Input: part model. Units: mm. Frame: model coordinates. Face numbers are marked on the shaded views. A direction names the side the tool comes from. Give positions to 0.01 mm unless a question says otherwise; leave off trailing zeros. Loops run counter-clockwise (first coordinate to the right, second up) from the corner with the lowest first, then second, coordinate; pieces in that order, holes last.
from build123d import *

# Parameters (mm, degrees)
SKETCH2_W            = 127
SKETCH2_H            = 406.4
BOSS_EXTRUDE1_DEPTH  = 3.175
SKETCH3_W            = 127
SKETCH3_H            = 3.175
BOSS_EXTRUDE2_DEPTH  = 127
FILLET1_R            = 3.175
SKETCH4_R            = 2.54
CUT_EXTRUDE1_DEPTH   = 429.448574802
SKETCH5_R            = 4.7625
SKETCH5_R_2          = 2.15
CUT_EXTRUDE2_DEPTH   = 248.894110458
CONVERT_SOLID1_START = -63.5
CONVERT_SOLID1_DEPTH = 127
FILLET2_R            = 2.54


# Read off the part's stored shape, not the designer's step: Convert-Solid1
with BuildPart() as part:
    # Sketch2 → Boss-Extrude1 (new body)
    with BuildSketch(Plane.XY):
        Rectangle(SKETCH2_W, SKETCH2_H)
    extrude(amount=BOSS_EXTRUDE1_DEPTH)

    # Sketch3 → Boss-Extrude2 (add)
    with BuildSketch(Plane.XY.offset(3.175)):
        with Locations((0, -201.6125)):
            Rectangle(SKETCH3_W, SKETCH3_H)
    extrude(amount=BOSS_EXTRUDE2_DEPTH)

    # Fillet1
    fillet1_edges = [part.edges().sort_by_distance(p)[0] for p in [
        (0, -200.025, 3.175),
        (0, -203.2, 0),
    ]]
    fillet(fillet1_edges, radius=FILLET1_R)

    # Sketch4 → Cut-Extrude1 (cut, through all)
    with BuildSketch(Plane(origin=(0, -200.025, 0), x_dir=(1, 0, 0), z_dir=(0, 1, 0))):
        with BuildLine():
            ThreePointArc((-6.167107762, -66.675), (0.182892238, -73.025), (6.532892238, -66.675))
            Line((6.532892238, -66.675), (6.532892238, -28.575))
            ThreePointArc((6.532892238, -28.575), (0.182892238, -22.225), (-6.167107762, -28.575))
            Line((-6.167107762, -28.575), (-6.167107762, -66.675))
        make_face()
        with Locations(Location((12.7, -79.375, 0), (0, 0, 270))):
            Circle(SKETCH4_R)
        with Locations(Location((50.8, -79.375, 0), (0, 0, 270))):
            Circle(SKETCH4_R)
        with Locations(Location((50.8, -15.875, 0), (0, 0, 270))):
            Circle(SKETCH4_R)
        with Locations(Location((12.7, -15.875, 0), (0, 0, 270))):
            Circle(SKETCH4_R)
    extrude(amount=-CUT_EXTRUDE1_DEPTH, mode=Mode.SUBTRACT)

    # Sketch5 → Cut-Extrude2 (cut, through all)
    with BuildSketch(Plane.XY.offset(3.175)):
        with Locations((-50.8, 187.96)):
            Circle(SKETCH5_R)
        with Locations((50.8, 187.96)):
            Circle(SKETCH5_R)
        with Locations((-50.8, -165.1)):
            Circle(SKETCH5_R)
        with Locations((50.8, -165.1)):
            Circle(SKETCH5_R)
        with Locations((34.20875, 175.39)):
            Circle(SKETCH5_R_2)
        with Locations((4.20875, 175.39)):
            Circle(SKETCH5_R_2)
        with Locations((4.20875, 145.69)):
            Circle(SKETCH5_R_2)
        with Locations((34.20875, 145.69)):
            Circle(SKETCH5_R_2)
    extrude(amount=-CUT_EXTRUDE2_DEPTH, mode=Mode.SUBTRACT)

    # Convert-Solid1 outline → Convert-Solid1 (cut)
    with BuildSketch(Plane.YZ.offset(CONVERT_SOLID1_START)):
        with BuildLine():
            ThreePointArc((-196.85, 1.5875), (-200.217596045, 2.982403955), (-201.6125, 6.35))
            Line((-201.6125, 6.35), (-201.6125, 130.175))
            Line((-201.6125, 130.175), (-203.2, 130.175))
            Line((-203.2, 130.175), (-203.2, 3.175))
            ThreePointArc((-203.2, 3.175), (-202.27006403, 0.92993597), (-200.025, 0))
            Line((-200.025, 0), (203.2, 0))
            Line((203.2, 0), (203.2, 1.5875))
            Line((203.2, 1.5875), (-196.85, 1.5875))
        make_face()
    extrude(amount=CONVERT_SOLID1_DEPTH, mode=Mode.SUBTRACT)

    # Fillet2
    fillet2_edges = [part.edges().sort_by_distance(p)[0] for p in [
        (63.5, -200.81875, 130.175),
        (-63.5, -200.81875, 130.175),
        (-63.5, 203.2, 2.38125),
        (63.5, 203.2, 2.38125),
    ]]
    fillet(fillet2_edges, radius=FILLET2_R)


solid = part.part
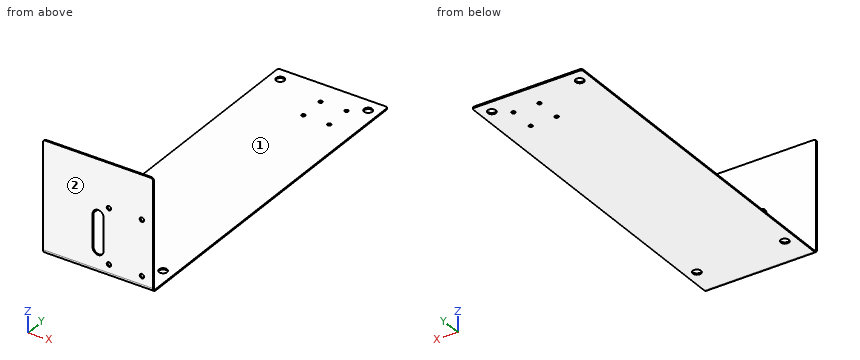
(1) Pin query (flat end, axial travel): pin 1 Ø1 at (x, y) = (-49.5, 13.5) entering from +Z (3 decimals); pin 2 Ø4.5 at (x, z) = (50.8, 79.375) entering from +Y; pin 3 Ø8 at (x, z) = (11.5, 39) entering from +Y (3 decimals). Return the tip coordinate at first contact, or that it passes through.
Values follow:
pin 1: stops at z = 3.175
pin 2: passes through
pin 3: stops at y = -200.025
(2) Cut plane C-C (x = -50.8). Count the separate pieces of the cut face and the enclosed holes in it, and give its area (3 significant figures).
Values follow:
separate pieces: 3
enclosed holes: 0
area: 811 mm2
(3) Cut plane B-B (z = 46.5). Return the cut outline in (x, y) (1 decimal), and give its area (3 significant figures).
Values follow:
outline: (-63.5, -201.6) - (-6.2, -201.6) - (-6.2, -200) - (-63.5, -200) - close; (6.5, -201.6) - (63.5, -201.6) - (63.5, -200) - (6.5, -200) - close
area: 181 mm2
(4) Cut plane A-A (y = -165.1). Return the cut outline in (x, z) (1 decimal), and give its area (3 significant figures).
Values follow:
outline: (-63.5, 1.6) - (-55.6, 1.6) - (-55.6, 3.2) - (-63.5, 3.2) - close; (-46, 1.6) - (46, 1.6) - (46, 3.2) - (-46, 3.2) - close; (55.6, 1.6) - (63.5, 1.6) - (63.5, 3.2) - (55.6, 3.2) - close
area: 171 mm2
(5) Reachability of the marked faces 1 and 2 from +Z, -Z, +X, -X, +Y, -Y: full face, straight path, thin tool, end or side. Return the list, or none.
Values follow:
face 1: +Z, +X, -X, +Y
face 2: +Z, -Z, +X, -X, -Y
(6) Ray query, probe 1 along X at (y, z) = (175.39, 2.25); probe 2 along Z at (x, y) = (12, -201) (3 decimals); probe 3 along Z at (x, y) = (43, -142) (1 decimal). Return the intervals inside material, ascending.
Values follow:
probe 1: x = -63.5 to 2.06, 6.36 to 32.06, 36.36 to 63.5
probe 2: z = 4.014 to 13.433, 18.317 to 76.933, 81.817 to 130.175
probe 3: z = 1.6 to 3.2
